Study the drawing (mm; zero at the part's minimum x, y, z) and answer. A direction names the side the tool comes from. Coordinates: 2 decimals unless noted, no trailing zeros. Loops run counter-clockwise (first coordinate to the right, second up) from the corner with the lowest first, then second, coordinate; pieces in that order, holes last. Notation, with made-up numbers: (48, -4) -> (58, -4) arc R31 cw to (58, 31) -> close; hole circle Ø6 at (-39, 74). An arc over 180 degrees is marked (long way). Answer as a JSON object with one key per item and string values. Group by question number.
Q1. Determine the mould class of the marked faces 1, 2, 3 and 4 for opening direction X: released by +X, released by -X, zero draft, split by the parting line, or undercut.
Q2. The part is cut by section C-C on z = 38. Write down the section's boundary in (x, y), and give its area (3 significant figures).
Q3. The part is cut by section D-D on y = 28. State how many separate pieces and enclosed holes the cut face has, and give its area (3 significant figures).
Q4. Straight lines are drawn through the part: line 1 along X through (y, z) = (105, 2.15); line 2 along Z through (x, y) = (109.9, 25); line 3 along X through (y, z) = (16.5, 60). For each, find the intervals that lie inside material, in ascending order. Write a range as [from, to].
Q5. The part is cut by section A-A on z = 27. Write down the section's boundary in (x, y).
Q6. The part is cut by section B-B on y = 103. Write down the section's boundary in (x, z).
Q7. Each of these flat-tipped pins is pushed along its axis until it touches: P1, Ø6, axis at x = 44.5, y = 38.5, coming from the +Z side; P2, Ø8, axis at y = 25, z = 62, coming from the -X side; P3, Ø2, axis at x = 85, y = 63, coming from the -Z side; P4, Ø2.5, axis at y = 97.5, z = 3.5, coming from the +X side. Where does it stop, or does it pass through?
Q8. For the marked faces 5 and 6, determine the directions among +Z, -Z, +X, -X, +Y, -Y from which every point of the face is accessible in a straight line to the end or side of a thin tool.
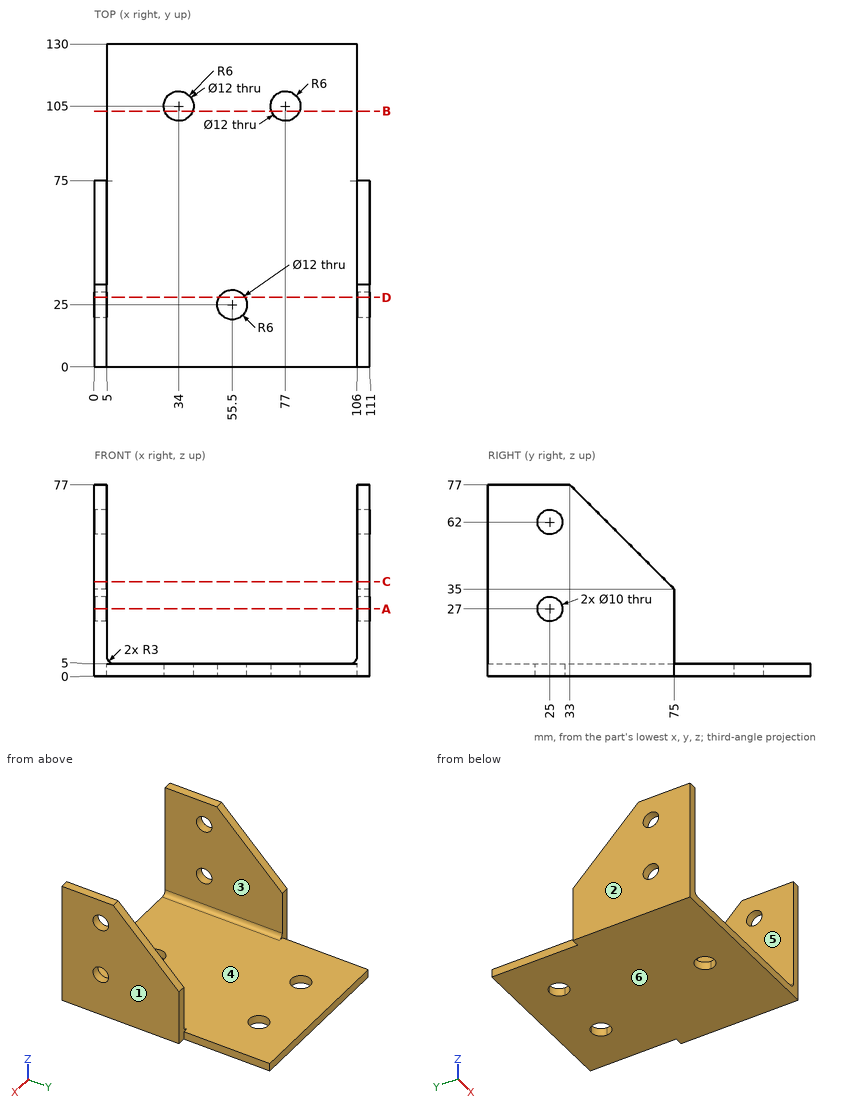
Final values:
{
 "1": {"face 1": "released by +X", "face 2": "released by -X", "face 3": "undercut", "face 4": "undercut"},
 "2": {"outline": "(0, 0) -> (5, 0) -> (5, 72) -> (0, 72) -> close; (106, 0) -> (111, 0) -> (111, 72) -> (106, 72) -> close", "area": "720 mm2"},
 "3": {"separate pieces": "6", "enclosed holes": "0", "area": "1,070 mm2"},
 "4": {"line 1": "x = [5, 28], [40, 71], [83, 106]", "line 2": "z = [0, 22], [32, 57], [67, 77]", "line 3": "x = [0, 5], [106, 111]"},
 "5": {"outline": "(0, 0) -> (5, 0) -> (5, 20) -> (0, 20) -> close; (0, 30) -> (5, 30) -> (5, 75) -> (0, 75) -> close; (106, 0) -> (111, 0) -> (111, 20) -> (106, 20) -> close; (106, 30) -> (111, 30) -> (111, 75) -> (106, 75) -> close"},
 "6": {"outline": "(5, 0) -> (28.34, 0) -> (28.34, 5) -> (5, 5) -> close; (39.66, 0) -> (71.34, 0) -> (71.34, 5) -> (39.66, 5) -> close; (82.66, 0) -> (106, 0) -> (106, 5) -> (82.66, 5) -> close"},
 "7": {"P1": "stops at z = 5", "P2": "passes through", "P3": "stops at z = 0", "P4": "stops at x = 106"},
 "8": {"face 5": "+Z, +Y, -Y", "face 6": "-Z, +X, -X, +Y, -Y"}
}
